from build123d import *

# Parameters (mm, degrees)
SKETCH1_W                                       = 146.05
SKETCH1_H                                       = 152.4
BOSS_EXTRUDE1_DEPTH                             = 12
F_1_4_CLEARANCE_HOLE1_D                         = 6.5278
SKETCH4_W                                       = 12
SKETCH4_H                                       = 3.11
CUT_EXTRUDE1_DEPTH                              = 170.417858046
CBORE_FOR_10_SOCKET_HEAD_CAP_SCREW1_D           = 4.9784
CBORE_FOR_10_SOCKET_HEAD_CAP_SCREW1_CBORE_D     = 9.525
CBORE_FOR_10_SOCKET_HEAD_CAP_SCREW1_CBORE_DEPTH = 4.826
LPATTERN1_COUNT                                 = 2
LPATTERN1_PITCH                                 = 44.958
LPATTERN1_COUNT_DIR2                            = 2
LPATTERN1_PITCH_DIR2                            = 60.132999876


with BuildPart() as part:
    # Sketch1 → Boss-Extrude1 (new body)
    with BuildSketch(Plane(origin=(0, 0, 0), x_dir=(1, 0, 0), z_dir=(0, 1, 0))):
        Rectangle(SKETCH1_W, SKETCH1_H)
    extrude(amount=-BOSS_EXTRUDE1_DEPTH)

    # 1/4 Clearance Hole1 (through all)
    with Locations(Plane(origin=(0, 0, 0), x_dir=(1, 0, 0), z_dir=(0, 1, 0))):
        with Locations((-36.195, 63.5), (-36.195, -38.1), (65.405, -38.1), (65.405, 63.5)):
            Hole(F_1_4_CLEARANCE_HOLE1_D / 2)

    # Sketch4 → Cut-Extrude1 (cut, through all)
    with BuildSketch(Plane.XY.offset(76.2)):
        with Locations((52.705, -1.555)):
            Rectangle(SKETCH4_W, SKETCH4_H)
    cut_extrude1 = extrude(amount=-CUT_EXTRUDE1_DEPTH, mode=Mode.SUBTRACT)

    # CBORE for #10 Socket Head Cap Screw1 (through all)
    with Locations(Plane(origin=(0, -12, 0), x_dir=(-1, 0, 0), z_dir=(0, -1, 0))):
        with Locations((-52.705, -63.5), (-52.705, 63.5), (-52.705, 0)):
            cbore_for_10_socket_head_cap_screw1 = CounterBoreHole(CBORE_FOR_10_SOCKET_HEAD_CAP_SCREW1_D / 2, CBORE_FOR_10_SOCKET_HEAD_CAP_SCREW1_CBORE_D / 2, CBORE_FOR_10_SOCKET_HEAD_CAP_SCREW1_CBORE_DEPTH)

    # LPattern1: Cut-Extrude1, CBORE for _10 Socket Head Cap Screw1 2 × 2
    with Locations(*[Vector(-1, 0, 0) * (i * LPATTERN1_PITCH) + Vector(-1, 0, 0) * (j * LPATTERN1_PITCH_DIR2) for i in range(LPATTERN1_COUNT) for j in range(LPATTERN1_COUNT_DIR2) if (i, j) != (0, 0)]):
        add(cut_extrude1, mode=Mode.SUBTRACT)
        add(cbore_for_10_socket_head_cap_screw1, mode=Mode.SUBTRACT)


solid = part.part
Model file for the job. Use its own axes, mm. A direction names the side the tool comes from. Coordinates: 2 decimals unless noted, no trailing zeros. Order: outer loops, then holes, each group sorted by start corner. A loop starts at its lowest first (then second) coordinate and runs counter-clockwise, first axis right, second up. Notation, with made-up numbers: M -8,58 L 27,58 A11 ccw 27,72 Z; hole C 36.5,12.25 d4. An arc over 180 degrees is marked long. Return JSON: item names as keys, results as strings.
1. Flat gauge pins, fed straight in: pin 1 (4 mm diameter, centred on x = 7.747, z = 0, fed in from -Y); pin 2 (5.5 mm diameter, centred on x = 7.747, z = -63.5, fed in from +Y); pin 3 (5 mm diameter, centred on x = 53.5, z = -62.5, fed in from -Y). Where does each tip first touch, or does it go through?
Ans:
{"pin 1": "through", "pin 2": "y = -3.11", "pin 3": "y = -7.17"}
2. Saw through at B-B (z = -63.5). Give the number of separate pieces and of enclosed holes in the cut face, and give its area (3 significant figures).
Ans:
{"separate pieces": "7", "enclosed holes": "0", "area": "1,180 mm^2"}
3. Pull direction X, two halves, no side cores. Call faces 1 (the face through (73.025, -6, 1)), 2 (the face through (-37.701, -6.084, 40.996)), 3 (the face through (30, 0, -1)): +X half, -X half, draft (parallel to the pull), parting line (faces both ways), or undercut.
Ans:
{"face 1": "+X half", "face 2": "undercut", "face 3": "draft"}
4. Saw through at A-A (z = 30). Give the cut face in (x, y) (3 decimals), and give its area (3 significant figures).
Ans:
{"outline": "M -73.025,-12 L 73.025,-12 L 73.025,0 L 58.705,0 L 58.705,-3.11 L 46.705,-3.11 L 46.705,0 L 13.747,0 L 13.747,-3.11 L 1.747,-3.11 L 1.747,0 L -1.428,0 L -1.428,-3.11 L -13.428,-3.11 L -13.428,0 L -46.386,0 L -46.386,-3.11 L -58.386,-3.11 L -58.386,0 L -73.025,0 Z", "area": "1,600 mm^2"}
5. Tool access for faces 4 (the face through (-9, -7.174, 66)), 5 (the face through (-30, 0, -1)), 6 (the face through (-55, -3.11, 1)): list every direction of +Z, -Z, +X, -X, +Y, -Y with a clear straight run to the whole face (end or side of a thin tool).
Ans:
{"face 4": "-Y", "face 5": "+Z, -Z, +X, -X, +Y", "face 6": "+Z, -Z, +Y"}
6. Drill centre lines: probe 1 along X at (y, z) = (-8.05, 63.5) (1 decimal); probe 2 along X at (y, z) = (-1, -29.5) (3 decimals); probe 3 along X at (y, z) = (-6.75, 38.1) (3 decimals). Where is each one in solid material? Low to high.
Ans:
{"probe 1": "-73 to -57.1, -47.6 to -12.2, -2.7 to 3, 12.5 to 47.9, 57.5 to 73", "probe 2": "-73.025 to -58.386, -46.386 to -13.428, -1.428 to 1.747, 13.747 to 46.705, 58.705 to 73.025", "probe 3": "-73.025 to -39.459, -32.931 to 62.141, 68.669 to 73.025"}
